Read the model definition and answer for the solid it produces. Units are mm, in the model's axes. Face numbers are marked on the shaded views. A direction names the side the tool comes from. Coordinates: 2 decimals unless noted, no trailing zeros. Write each loop counter-clockwise with the first axis right and the second up, starting at its lowest first coordinate (ties: lowest second). Pieces come first, ordered by that corner, then holes. Notation, with made-up numbers: (22.25, 14.5) -> (49.25, 14.5) arc R7 ccw to (49.25, 19.5) -> close; hole circle Ø8 at (48, -32). An arc over 180 degrees is marked (long way). Answer as a JSON object with one key per item and string values. Group by question number.
(1) Find section B-B (y = 26). Give the vertices of the cut face in (x, z).
(2) Find section C-C (x = 3). Give the vertices of the cut face in (y, z).
(3) Straight lines are drawn through the part: L1, parallel to X at y = 18, z = -2; L2, parallel to Y at x = -12, z = 7; L3, parallel to Y at x = -2, z = -0.75. For each, find the intervals that lie inside material, in ascending order.
(4) Find section D-D (z = -10.5). Give the vertices of the cut face in (x, y).
(5) Which of the six approach directions +Z, -Z, +X, -X, +Y, -Y give full straight-line access (tool end or side, diameter ignored) to the marked faces 1, 2 and 3?
(6) Flat-ended cylindrical pins translate along their axes: P1, Ø0.9, axis at x = 0, z = 3, coming from the -Y side; P2, Ø6.5, axis at x = 6, y = -7.5, coming from the +Z side; P3, Ø2, axis at y = 16, z = -11, coming from the +X side. Find the tip coordinate at first contact, or state that the pin passes through.
(7) Find section A-A (x = 13.5). Give the vertices of the cut face in (y, z).
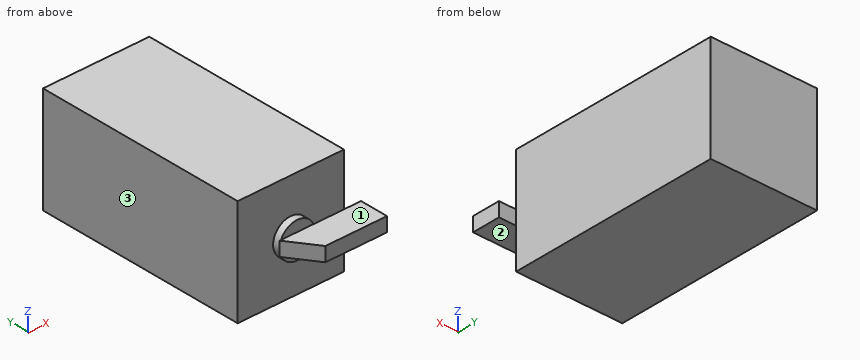
from build123d import *

# Parameters (mm, degrees)
SKETCH1_W                = 30
SKETCH1_H                = 30
BOSS_EXTRUDE1_DEPTH      = 60
SKETCH2_R                = 5
BOSS_EXTRUDE2_DEPTH      = 2
BOSS_EXTRUDE3_DEPTH      = 2
BOSS_EXTRUDE3_DEPTH_BACK = 2


with BuildPart() as part:
    # Sketch1 → Boss-Extrude1 (new body)
    with BuildSketch(Plane(origin=(0, 0, 0), x_dir=(1, 0, 0), z_dir=(0, 1, 0))):
        Rectangle(SKETCH1_W, SKETCH1_H)
    extrude(amount=BOSS_EXTRUDE1_DEPTH)

    # Sketch2 → Boss-Extrude2 (add)
    with BuildSketch(Plane.XZ):
        Circle(SKETCH2_R)
    extrude(amount=BOSS_EXTRUDE2_DEPTH)

    # Sketch4 → Boss-Extrude3 (add, two sides)
    with BuildSketch(Plane.XY) as boss_extrude3_sk:
        Polygon((-5, -2), (18, -2), (18, -10), (0.601660306, -10), align=None)
    extrude(amount=BOSS_EXTRUDE3_DEPTH)
    extrude(boss_extrude3_sk.sketch, amount=-BOSS_EXTRUDE3_DEPTH_BACK)


solid = part.part
Results below:
{
 "1": {"outline": "(-15, -15) -> (15, -15) -> (15, 15) -> (-15, 15) -> close"},
 "2": {"outline": "(-10, -2) -> (-2, -2) -> (-2, -4) -> (0, -4) -> (0, -15) -> (60, -15) -> (60, 15) -> (0, 15) -> (0, 4) -> (-2, 4) -> (-2, 2) -> (-10, 2) -> close"},
 "3": {"L1": "x = -15 to 15", "L2": "y = 0 to 60", "L3": "y = -6.28 to 60"},
 "4": {"outline": "(-15, 0) -> (15, 0) -> (15, 60) -> (-15, 60) -> close"},
 "5": {"face 1": "+Z, +X, -X, -Y", "face 2": "-Z, +X, -X, -Y", "face 3": "+Z, -Z, -X, +Y, -Y"},
 "6": {"P1": "stops at y = -2", "P2": "stops at z = 2", "P3": "stops at x = 15"},
 "7": {"outline": "(-10, -2) -> (-2, -2) -> (-2, 2) -> (-10, 2) -> close; (0, -15) -> (60, -15) -> (60, 15) -> (0, 15) -> close"}
}
